Build history of the part. All positions in model axes, mm. Face numbers are marked on the shaded views. Give positions to 0.01 mm unless a question says otherwise; leave off trailing zeros. Order: outer loops, then holes, each group sorted by start corner. A loop starts at its lowest first (then second) coordinate and runs counter-clockwise, first axis right, second up. Notation, with made-up numbers: (13.25, 15) - (54.25, 15) arc R11 ccw to (54.25, 34) - close; hole circle Ø7 at (73, 80.25). An arc over 180 degrees is marked (long way). Use a Markdown table: item, result. Add a question column.
(1) Wall check: line 1 (Y direction, x = -1.35, z = 1.1); line 2 (Y direction, x = -2.45, z = 1.6); line 3 (X direction, y = -1, z = 1). Give the ranges that are in metal, low to high.
(2) Slice it at B-B (z = 0.75). Write the cut outline in (x, y), then the cut area to 3 significant figures.
(3) Slice it at A-A (x = 0). Write the cut outline in (y, z).
(4) Flat gauge pin, fed straight in: pin 1 (1 mm diameter, centred on x = -1.5, z = 1, fed in from -Y). Where does the tip first touch, or does it go through?
(5) Mould opens along Y. For the marked faces 1, 2 and 3 say: +Y half, -Y half, draft (parallel to the pull), parting line (faces both ways), or undercut.
(6) Slice it at C-C (z = 0.2). Write the cut outline in (x, y), then the cut area to 3 significant figures.
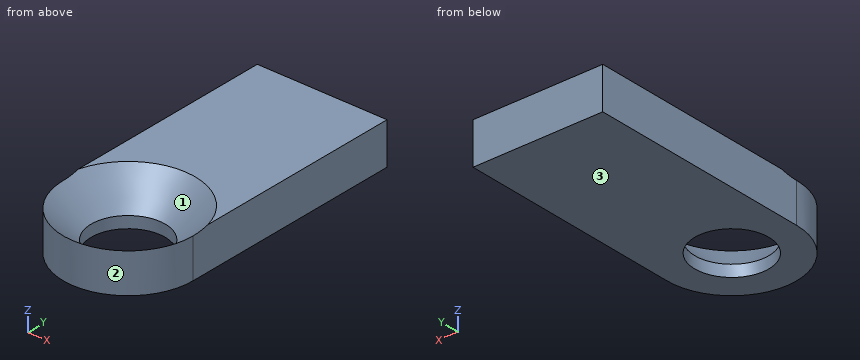
Autodesk Inventor part; units mm, degrees
ref_plane "YZ Plane" through (0, 0, 0) normal (1, 0, 0) x (0, 1, 0)
ref_plane "XZ Plane" through (0, 0, 0) normal (0, 1, 0) x (-1, 0, 0)
ref_plane "XY Plane" through (0, 0, 0) normal (0, 0, 1) x (1, 0, 0)
sketch "Sketch1" plane through (0, 0, 0) normal (0, 0, 1) x (1, 0, 0)
  arc A0 (-2.8, 0) -> (2.8, 0) centre (0, 0) ccw
  circle A1 centre (0, 0) radius 1.6
  line L0 (-2.8, 0) -> (-2.8, 9.8)
  line L1 (-2.8, 9.8) -> (2.8, 9.8)
  line L2 (2.8, 9.8) -> (2.8, 0)
  dimension "d0" = 3.2
  dimension "d1" = 2.8
  dimension "d2" = 9.8
extrude "Extrusion1" add sketch "Sketch1" along normal blind 1.8
chamfer "Chamfer1" distance 1.3 angle 45 1 edges at (-1.6, 0, 1.8)
Solution:
| question | item | result |
|---|---|---|
| 1 | line 1 | -2.45 to -1.74, 1.74 to 9.8 |
| 1 | line 2 | -1.36 to -1.13, 1.13 to 9.8 |
| 1 | line 3 | -2.62 to -1.85, 1.85 to 2.62 |
| 2 | outline | (-2.8, 0) arc R2.8 ccw to (2.8, 0) - (2.8, 9.8) - (-2.8, 9.8) - close; hole circle Ø3.7 at (0, 0) |
| 2 | area | 56.4 mm2 |
| 3 | outline | (-2.8, 0) - (-1.6, 0) - (-1.6, 0.5) - (-2.8, 1.7) - close; (1.6, 0) - (9.8, 0) - (9.8, 1.8) - (2.9, 1.8) - (1.6, 0.5) - close |
| 4 | pin 1 | y = -2.62 |
| 5 | face 1 | undercut |
| 5 | face 2 | -Y half |
| 5 | face 3 | draft |
| 6 | outline | (-2.8, 0) arc R2.8 ccw to (2.8, 0) - (2.8, 9.8) - (-2.8, 9.8) - close; hole circle Ø3.2 at (0, 0) |
| 6 | area | 59.2 mm2 |
